Verification items for this drawing (mm, ordinates from the low corner). A direction names the side the tool comes from. Coordinates: 2 decimals unless noted, no trailing zeros. Write each loop counter-clockwise with the first axis right and the second up, starting at its lowest first coordinate (ties: lowest second). Pieces come first, ordered by that corner, then holes. Notation, with made-up numbers: M 29,26 L 53,26 A12 ccw 53,42 Z; hole C 80,-33 d9. An arc over 180 degrees is marked long. Put each result on its own line as item: value. Start each with the question number.
1) Cross-section at D-D on z = 21. Record the cut outline in (x, y), plus the area to 3 significant figures.
2) Cross-section at A-A on z = 15.5. Record the cut outline in (x, y), plus the area to 3 significant figures.
3) Cross-section at C-C on z = 1.75. Record the cut outline in (x, y).
4) Cross-section at B-B on x = 27.5. Record the cut outline in (y, z), plus the area to 3 significant figures.
5) Gauge pin test, flat end, axial feed: pin 1 (3 mm diameter, centred on y = 9.5, z = 20, fed in from +X). Record the tip position at first contact, or that the pin passes through.
6) Set-up check for the marked faces 1 and 2: record each of +Z, -Z, +X, -X, +Y, -Y from which the full face is reachable in a straight line by a thin tool's end or side.
7) Scan lines: line 1 along X through (y, z) = (8.5, 16); line 2 along X through (y, z) = (1.75, 4.5); line 3 along Z through (x, y) = (25.5, 8.5). Record each from-to range of solid material in increasing order.
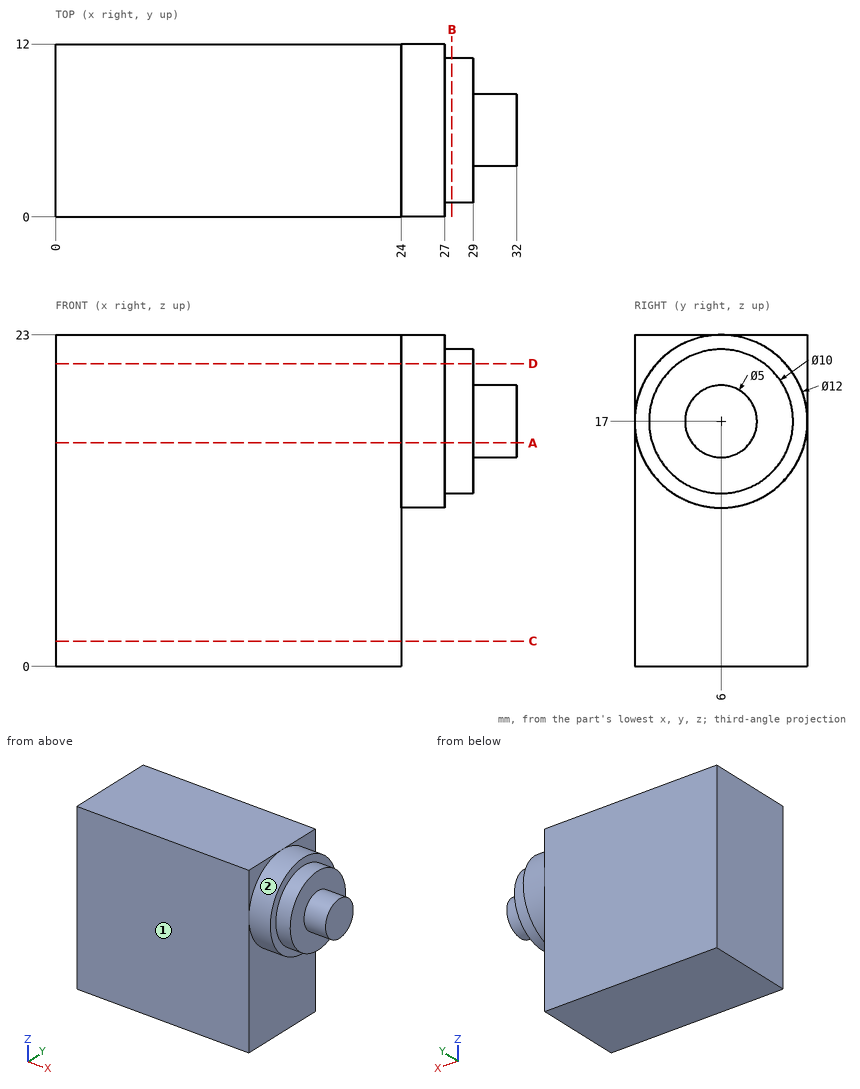
Answer key:
1. outline: M 0,0 L 24,0 L 24,1.53 L 27,1.53 L 27,3 L 29,3 L 29,9 L 27,9 L 27,10.47 L 24,10.47 L 24,12 L 0,12 Z
1. area: 327 mm²
2. outline: M 0,0 L 24,0 L 24,0.19 L 27,0.19 L 27,1.23 L 29,1.23 L 29,4 L 32,4 L 32,8 L 29,8 L 29,10.77 L 27,10.77 L 27,11.81 L 24,11.81 L 24,12 L 0,12 Z
2. area: 354 mm²
3. outline: M 0,0 L 24,0 L 24,12 L 0,12 Z
4. outline: C 6,17 d10
4. area: 78.5 mm²
5. pin 1: stops at x = 29
6. face 1: +Z, -Z, +X, -X, -Y
6. face 2: +X
7. line 1: x = 0 to 29
7. line 2: x = 0 to 24
7. line 3: z = 11.55 to 22.45
